Answer from the drawing. Dimensions are ordinates in mm from the lowest x, y and z of the part. A direction names the side the tool comes from. Give positions to 0.01 mm unless a question says otherwise; leave off trailing zeros. Write each loop counter-clockwise with the first axis right and the second up, starting at its lowest first coordinate (ties: lowest second). Pieces come first, ordered by that corner, then holes. Notation, with made-up numbers: M 45.25,49 L 102.25,49 A23 ccw 102.25,87 Z; hole C 52.5,10 d1. An arc over 180 degrees is marked long. Write each question's results on one line, items separated by ' | '. Start each with the question number.
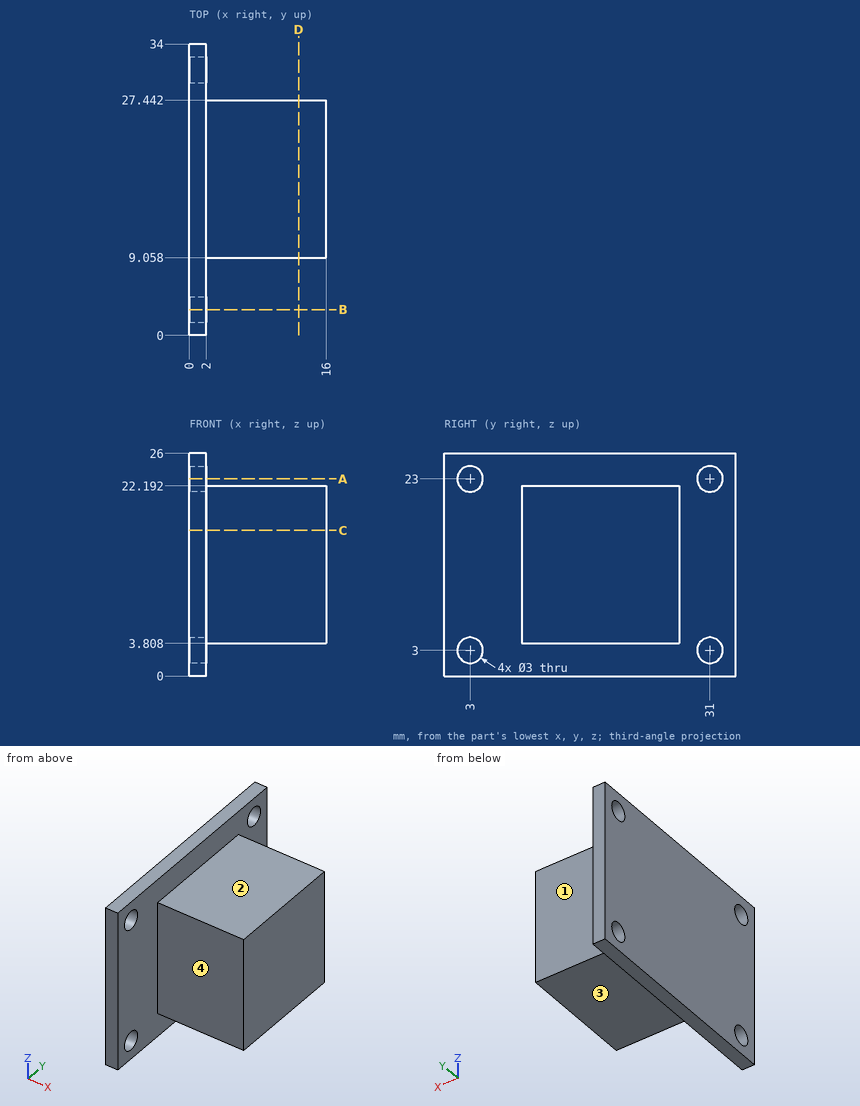
Item 1: Section D-D, the plane x = 12.75 is taken. Determine the outline of the cut face in (y, z).
Item 2: Straight lines are drawn through the part: line 1 (Y direction, x = 0.75, z = 23); line 2 (Z direction, x = 5.5, y = 11); line 3 (X direction, y = 3.5, z = 18.5). For each, find the intervals that lie inside material, in ascending order.
Item 3: Given P1, Ø4, axis at y = 31, z = 3, coming from the +X side; P2, Ø5, axis at y = 3, z = 3, coming from the -X side; P3, Ø3, axis at x = 10.5, z = 11, coming from the +Y side; P4, Ø7, axis at x = 12, y = 14, coming from the -Z side, each flat-ended and moving along its own axis, determine where each tip first touches the part or whether it passes through.
Item 4: Section A-A, the plane z = 23 is taken. Determine the outline of the cut face in (x, y).
Item 5: Section B-B, the plane y = 3 is taken. Determine the outline of the cut face in (x, z), then the cut area to 3 significant figures.
Item 6: Section C-C, the plane z = 17 is taken. Determine the outline of the cut face in (x, y), then the cut area to 3 significant figures.
Item 7: For the marked faces 1, 2, 3 and 4, determine the directions among +Z, -Z, +X, -X, +Y, -Y from which every point of the face is accessible in a straight line to the end or side of a thin tool.
Worked out:
1) outline: M 9.06,3.81 L 27.44,3.81 L 27.44,22.19 L 9.06,22.19 Z
2) line 1: y = 0 to 1.5, 4.5 to 29.5, 32.5 to 34 | line 2: z = 3.81 to 22.19 | line 3: x = 0 to 2
3) P1: stops at x = 2 | P2: stops at x = 0 | P3: stops at y = 27.44 | P4: stops at z = 3.81
4) outline: M 0,0 L 2,0 L 2,1.5 L 0,1.5 Z; M 0,4.5 L 2,4.5 L 2,29.5 L 0,29.5 Z; M 0,32.5 L 2,32.5 L 2,34 L 0,34 Z
5) outline: M 0,0 L 2,0 L 2,1.5 L 0,1.5 Z; M 0,4.5 L 2,4.5 L 2,21.5 L 0,21.5 Z; M 0,24.5 L 2,24.5 L 2,26 L 0,26 Z | area: 40.0 mm²
6) outline: M 0,0 L 2,0 L 2,9.06 L 16,9.06 L 16,27.44 L 2,27.44 L 2,34 L 0,34 Z | area: 325 mm²
7) face 1: +Z, -Z, +X, +Y | face 2: +Z, +X, +Y, -Y | face 3: -Z, +X, +Y, -Y | face 4: +Z, -Z, +X, -Y
